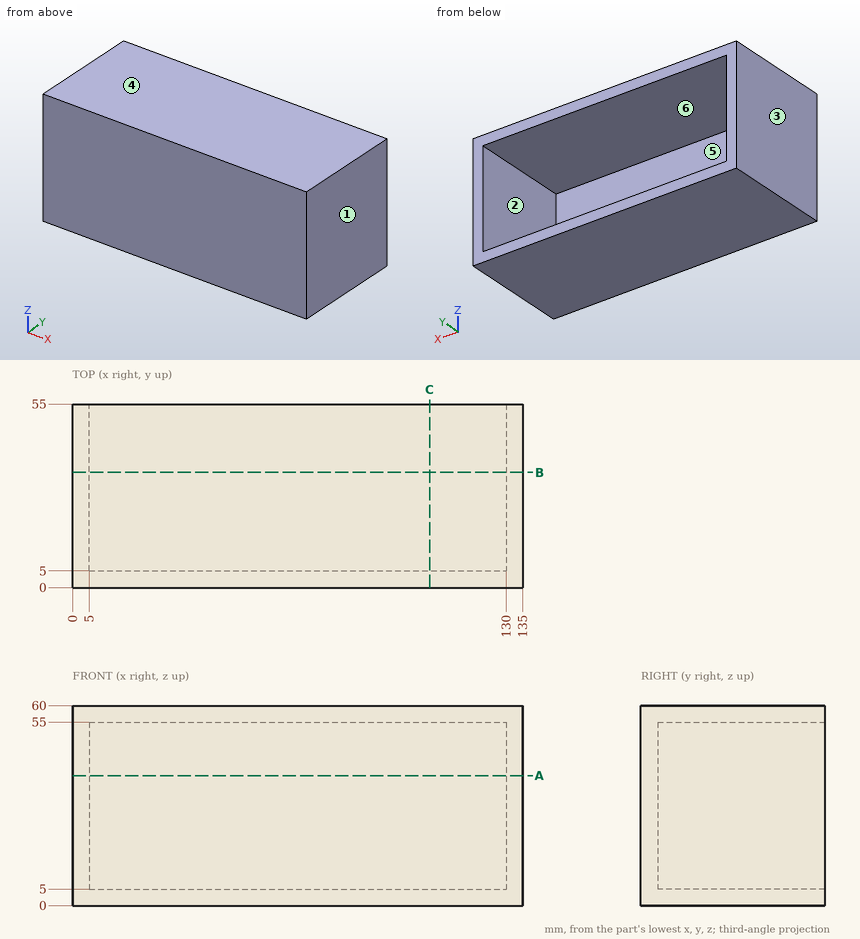
Design review of the part shown in the three views and the two pictorial views. Dimensions are in mm from the part's minimum x, y and z. A direction names the side the tool comes from. Coordinates: 2 decimals unless noted, no trailing zeros. Order: outer loops, then holes, each group sorted by start corner. A loop starts at its lowest first (then second) coordinate and runs counter-clockwise, first axis right, second up.
Item 1: Take a section at B-B, the plane y = 34.5. Write out the cut boundary in (x, z).
Item 2: Take a section at A-A, the plane z = 39. Write out the cut boundary in (x, y).
Item 3: For the marked faces 1 and 2, list the 3-axis set-ups (+Z, -Z, +X, -X, +Y, -Y) from which the entire face can be reached by the end or side of a thin tool; tool diameter is ignored.
Item 4: The part is to be moulded in two halves that separate along X. For the marked faces 3, 4, 5 and 6, say which applies: pulls with the +X half, pulls with the -X half, needs draft (parallel to the pull), parting line crosses it, or undercut.
Item 5: For line 1 (X direction, y = 46.5, z = 32); line 2 (Z direction, x = 75, y = 52.5); line 3 (Y direction, x = 43.5, z = 25), list the stretches that pass through material, from the lowest coordinate up.
Item 6: Take a section at C-C, the plane x = 107. Write out the cut boundary in (y, z).
The answers:
1. outline: (0, 0) - (135, 0) - (135, 60) - (0, 60) - close; hole (5, 5) - (130, 5) - (130, 55) - (5, 55) - close
2. outline: (0, 0) - (135, 0) - (135, 55) - (130, 55) - (130, 5) - (5, 5) - (5, 55) - (0, 55) - close
3. face 1: +Z, -Z, +X, +Y, -Y
3. face 2: +Y
4. face 3: pulls with the -X half
4. face 4: needs draft
4. face 5: undercut
4. face 6: undercut
5. line 1: x = 0 to 5, 130 to 135
5. line 2: z = 0 to 5, 55 to 60
5. line 3: y = 0 to 5
6. outline: (0, 0) - (55, 0) - (55, 5) - (5, 5) - (5, 55) - (55, 55) - (55, 60) - (0, 60) - close
